Geometry check sheet. Reference: drawing and pictorial views, mm from the part's lowest x, y, z. Coordinates: 2 decimals unless noted, no trailing zeros. Loops run counter-clockwise (first coordinate to the right, second up) from the corner with the lowest first, then second, coordinate; pieces in that order, holes last.
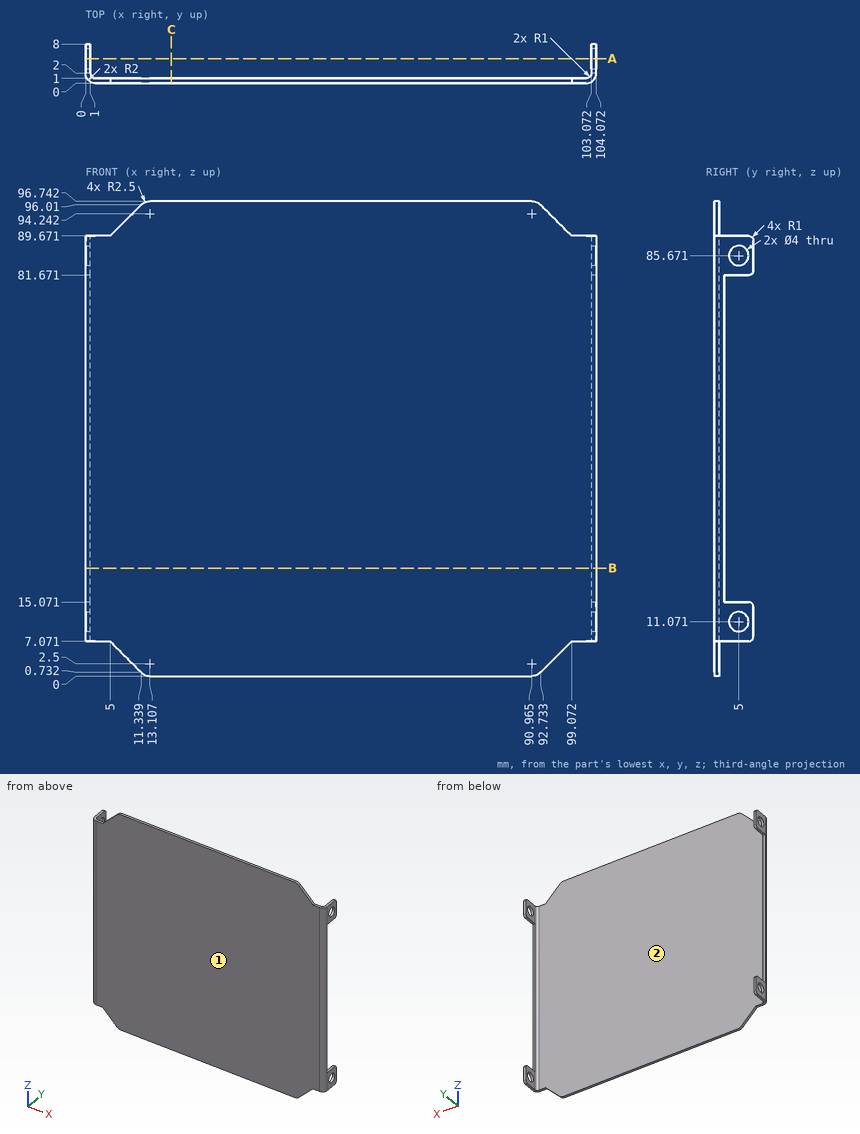
1) Mould release check, pull along X, two halves, no side actions. Record for the marked faces 1 and 2: +X half, -X half, draft (parallel to the pull), parting line (faces both ways), or undercut.
Data:
face 1: draft
face 2: undercut
2) Material ranges on probe 1 along Z at (x, y) = (0.3, 5); probe 2 along X at (y, z) = (4.5, 88.5); probe 3 along Y at (x, z) = (29, 37.5), recorded low to high.
Data:
probe 1: z = 7.07 to 9.07, 13.07 to 15.07, 81.67 to 83.67, 87.67 to 89.67
probe 2: x = 0 to 1, 103.07 to 104.07
probe 3: y = 0 to 1
3) Section check A-A on y = 5. Count the separate pieces of the cut face and the enclosed holes in it, and give its area (3 significant figures).
Data:
separate pieces: 8
enclosed holes: 0
area: 16.0 mm2
4) Depth check by flat-ended pin: pin 1 (1.8 mm diameter, centred on y = 4.5, z = 84.5, fed in from -X); pin 2 (4 mm diameter, centred on x = 102, y = 2.5, fed in from +Z); pin 3 (0.5 mm diameter, centred on x = 103.5, z = 53, fed in from +Y); pin 4 (4 mm diameter, centred on x = 52.5, z = 39, fed in from +Y). Enter the tip coordinate at first touch or a pass-through.
Data:
pin 1: stops at x = 0
pin 2: stops at z = 89.67
pin 3: stops at y = 2
pin 4: stops at y = 1
5) Section check C-C on x = 17.5. Record the cut outline in (y, z).
Data:
outline: (0, 0) - (1, 0) - (1, 96.74) - (0, 96.74) - close
6) Section check B-B on z = 22. Record the cut outline in (x, y).
Data:
outline: (0, 2) arc R2 ccw to (2, 0) - (102.07, 0) arc R2 ccw to (104.07, 2) - (103.07, 2) arc R1 cw to (102.07, 1) - (2, 1) arc R1 cw to (1, 2) - close
